from build123d import *

# Parameters (mm, degrees)
SKETCH1_R           = 2
BOSS_EXTRUDE1_DEPTH = 5
SKETCH2_R           = 7.5
BOSS_EXTRUDE2_DEPTH = 15
BOSS_EXTRUDE3_DEPTH = 15
FILLET1_R           = 1


with BuildPart() as part:
    # Sketch1 → Boss-Extrude1 (new body)
    with BuildSketch(Plane.XY):
        Circle(SKETCH1_R)
    extrude(amount=BOSS_EXTRUDE1_DEPTH)

    # Sketch2 → Boss-Extrude2 (add)
    with BuildSketch(Plane.XY.offset(5)):
        Circle(SKETCH2_R)
    extrude(amount=BOSS_EXTRUDE2_DEPTH)

    # Sketch3 → Boss-Extrude3 (add)
    with BuildSketch(Plane.XY.offset(20)):
        Polygon((-5.249682076, -5.356382931), (-10.321706995, -15.355132011), (10.321706995, -15.355132011), (5.249682076, -5.356382931), align=None)
    extrude(amount=-BOSS_EXTRUDE3_DEPTH)

    # Fillet1
    fillet1_edges = [part.edges().sort_by_distance(p)[0] for p in [
        (10.321706995, -15.355132011, 12.5),
        (-10.321706995, -15.355132011, 12.5),
    ]]
    fillet(fillet1_edges, radius=FILLET1_R)


solid = part.part
Read the model definition and answer for the solid it produces. Units are mm, in the model's axes. A direction names the side the tool comes from. Round coordinates to 2 decimals unless told otherwise and drop trailing zeros. Loops run counter-clockwise (first coordinate to the right, second up) from the corner with the lowest first, then second, coordinate; pieces in that order, holes last.
Q1. Each of these flat-tipped pins is pushed along its axis until it touches: pin 1 (12 mm diameter, centred on y = -4.5, z = 15, fed in from +X); pin 2 (5 mm diameter, centred on y = -6, z = 18, fed in from -X); pin 3 (12 mm diameter, centred on y = 5, z = 17, fed in from -X). Where does it stop, or does it pass through?
Q2. Consider probe 1 along Z at (x, y) = (-6.5, 1); probe 2 along Y at (x, z) = (-6, 7.5); probe 3 along X at (y, z) = (0.5, 13.75). Determine where each line is inside the solid, lowest interval first.
Q3. Which of the six approach directions +Z, -Z, +X, -X, +Y, -Y give full straight-line access (tool end or side, diameter ignored) to faces 1 (the face through (7.45, -9.69, 12.6)), 2 (the face through (0, -2, 2)), 3 (the face through (0, -4, 20))?
Q4. Section A-A on x = 0 is taken. Write down the section's boundary in (y, z), and give its area (3 significant figures).
Q5. Determine the mould class of faces 4 (the face through (-7.387, -9.57, 12.605)), 5 (the face through (0, -15.355, 13)), 6 (the face through (0, 0, 0)) for opening direction Y: released by +Y, released by -Y, zero draft, split by the parting line, or undercut.
Q6. Section C-C on y = 0 is taken. Write down the section's boundary in (x, z).
Q7. Section B-B on z = 8.5 is taken. Write down the section's boundary in (x, y), and give its area (3 significant figures).
Q8. Section D-D on y = -8.25 is taken. Write down the section's boundary in (x, z), and give its area (3 significant figures).
Output:
1. pin 1: stops at x = 7.86
1. pin 2: stops at x = -6.84
1. pin 3: stops at x = -7.5
2. probe 1: z = 5 to 20
2. probe 2: y = -15.36 to -6.84, -4.5 to 4.5
2. probe 3: x = -7.48 to 7.48
3. face 1: +Z, -Z, +X
3. face 2: -Z
3. face 3: +Z, +X, -X, +Y, -Y
4. outline: (-15.36, 5) - (-2, 5) - (-2, 0) - (2, 0) - (2, 5) - (7.5, 5) - (7.5, 20) - (-15.36, 20) - close
4. area: 363 mm2
5. face 4: undercut
5. face 5: released by -Y
5. face 6: zero draft
6. outline: (-7.5, 5) - (-2, 5) - (-2, 0) - (2, 0) - (2, 5) - (7.5, 5) - (7.5, 20) - (-7.5, 20) - close
7. outline: (-9.58, -13.9) arc R1 ccw to (-8.69, -15.36) - (8.69, -15.36) arc R1 ccw to (9.58, -13.9) - (5.25, -5.36) arc R7.5 ccw (long way) to (-5.25, -5.36) - close
7. area: 316 mm2
8. outline: (-6.72, 5) - (6.72, 5) - (6.72, 20) - (-6.72, 20) - close
8. area: 202 mm2
